Part model, mm, in its own coordinate system. Round coordinates to 2 decimals unless told otherwise and drop trailing zeros. Write each loop counter-clockwise with the first axis right and the second up, starting at its lowest first coordinate (ties: lowest second). Pieces come first, ordered by that corner, then holes. Notation, with made-up numbers: M -17,-15 L 32,-15 A7 ccw 32,-8 Z; hole C 78.25,60.5 d7. An arc over 180 degrees is marked long. Use a Markdown table: item, result. Add a question column.
1) Wall check: probe 1 along Z at (x, y) = (0, -175); probe 2 along Y at (x, z) = (7.75, 5); probe 3 along X at (y, z) = (-432, 1.25). Give the ranges that are in metal, low to high.
2) Slice it at A-A on y = -541.5. Write the cut outline in (x, z), plus the area to 3 significant figures.
3) Drop flat-ended pins along their axis: P1, Ø8, axis at x = 5.5, y = -227, coming from the +Z side; P2, Ø4, axis at y = -139, z = -3, coming from the +X side; P3, Ø12, axis at x = -6, y = -545, coming from the -Z side. Give the stop position or say it passes through.
```python
from build123d import *

# Parameters (mm, degrees)
F0_R     = 7
F0_R_2   = 3.81
F1_DEPTH = 630
F2_R     = 10
F2_R_2   = 7
F2_R_3   = 3.81
F3_DEPTH = 40
F4_W     = 4.28
F4_H     = 4.36


with BuildPart() as f1:
    # F0 (on Front) → F1 (new body)
    with BuildSketch(Plane.XZ):
        Circle(F0_R)
        Circle(F0_R_2, mode=Mode.SUBTRACT)
    extrude(amount=F1_DEPTH)

    # F2 (on face) → F3 (join)
    with BuildSketch(Plane(origin=(0, 0, 0), x_dir=(-1, 0, 0), z_dir=(0, 1, 0))):
        Circle(F2_R)
        Circle(F2_R_2, mode=Mode.SUBTRACT)
        Circle(F2_R_2)
        Circle(F2_R_3, mode=Mode.SUBTRACT)
    extrude(amount=F3_DEPTH)

    # F4 (on Right) → F5 (revolve, cut)
    with BuildSketch(Plane.YZ):
        with Locations((2.14, 2.18)):
            Rectangle(F4_W, F4_H)
        Polygon((4.28, 4.36), (4.28, 0), (11.98, 0), (11.98, 5.765), align=None)
        Polygon((11.98, 5.765), (11.98, 0), (47.75, 0), (47.75, 5.98), align=None)
    revolve(axis=Axis((0, 29.865, 0), (0, 1, 0)), mode=Mode.SUBTRACT)


solid = f1.part
```
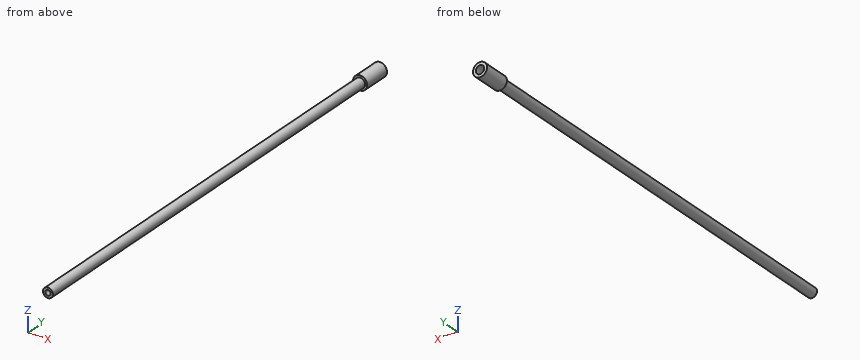
Entries:
| question | item | result |
|---|---|---|
| 1 | probe 1 | z = -7 to -3.81, 3.81 to 7 |
| 1 | probe 2 | y = 0 to 40 |
| 1 | probe 3 | x = -6.89 to -3.6, 3.6 to 6.89 |
| 2 | outline | C 0,0 d14; hole C 0,0 d7.62 |
| 2 | area | 108 mm^2 |
| 3 | P1 | stops at z = 6.84 |
| 3 | P2 | stops at x = 6.93 |
| 3 | P3 | stops at z = -7 |
